Input: part model. Units: mm. Frame: model coordinates. Face numbers are marked on the shaded views. A direction names the side the tool comes from. Coordinates: 2 decimals unless noted, no trailing zeros. Write each loop counter-clockwise with the first axis right and the second up, starting at its lowest first coordinate (ties: lowest second). Pieces come first, ordered by that corner, then holes. Notation, with made-up numbers: M 8.5,67 L 19.5,67 A23 cw 19.5,97 Z; hole C -21.75,75 d2. An arc over 180 degrees is marked long. Use one line per item in the form item = value.
Solid Edge part; units mm, degrees
sketch "Sketch1" plane through (0, 0, 0) normal (0, 0, 1) x (1, 0, 0)
  arc A0 (60, 30) -> (60, -30) centre (60, 0) cw
  line L0 (0, -30) -> (60, -30)
  line L1 (-60, -30) -> (0, -30)
  arc A1 (-60, -30) -> (-60, 30) centre (-60, 0) cw
  line L2 (-60, 30) -> (0, 30)
  line L3 (0, 30) -> (60, 30)
  arc A2 (60, 15) -> (60, -15) centre (60, 0) cw
  line L4 (0, -15) -> (60, -15)
  line L5 (-60, -15) -> (0, -15)
  arc A3 (-60, -15) -> (-60, 15) centre (-60, 0) cw
  line L6 (-60, 15) -> (0, 15)
  line L7 (0, 15) -> (60, 15)
extrude "ExtrudedProtrusion_1" add sketch "Sketch1" along normal blind 20
sketch "Sketch2" plane through (0, 30, 10) normal (0, 1, 0) x (-1, 0, 0)
  circle A0 centre (0, 0) radius 5
extrude "ExtrudedProtrusion_2" add sketch "Sketch2" along normal blind 197
mirror "Mirror1" about plane through (0, 0, 10) normal (0, 1, 0) of "ExtrudedProtrusion_2"
sketch "Sketch3" plane through (0, -227, 10) normal (0, -1, 0) x (0, 0, -1)
  circle A0 centre (0, 0) radius 20
extrude "ExtrudedProtrusion_3" add sketch "Sketch3" along normal blind 40
mirror "Mirror2" about plane through (0, 0, 0) normal (0, -1, 0) of "ExtrudedProtrusion_3"
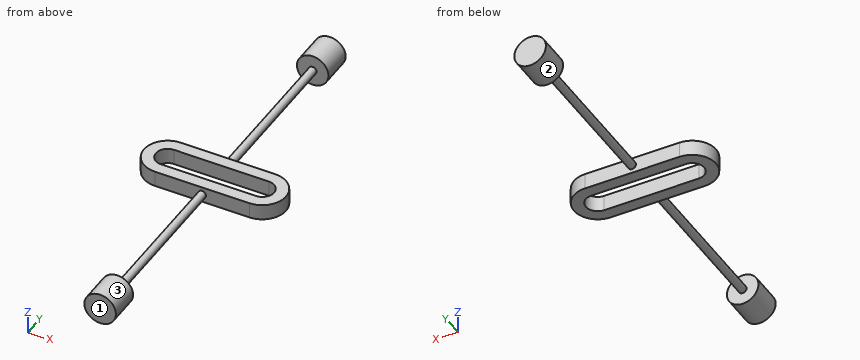
(1) Line query: probe 1 along Y at (x, z) = (10, 26); probe 2 along Y at (x, z) = (8.5, 0.5); probe 3 along Y at (x, z) = (52, 8). Output: solid intervals per line, ascending.
Computed:
probe_1 = -267 to -227, 227 to 267
probe_2 = -267 to -227, -30 to -15, 15 to 30, 227 to 267
probe_3 = -30 to -15, 15 to 30
(2) First-contact query: pin 1 Ø5 at (y, z) = (-152.5, 4.5) entering from -X; pin 2 Ø6 at (x, z) = (-24, 8.5) entering from -Y; pin 3 Ø10 at (x, z) = (21, 6.5) entering from +Y; pin 4 Ø1.5 at (x, z) = (-52.5, 17.5) entering from +Y. Flat tips, straight axial feed; report the tip coordinate or a pass-through.
Computed:
pin_1 = -4
pin_2 = -30
pin_3 = 267
pin_4 = 30
(3) Section query B-B on y = 0. Return the cut outline in (x, z), plus the area to 3 significant figures.
Computed:
outline = M -90,0 L -75,0 L -75,20 L -90,20 Z; M 75,0 L 90,0 L 90,20 L 75,20 Z
area = 600 mm^2
(4) Section query C-C on x = -38. Return the cut outline in (y, z).
Computed:
outline = M -30,0 L -15,0 L -15,20 L -30,20 Z; M 15,0 L 30,0 L 30,20 L 15,20 Z
(5) Section query A-A on x = 0. Return the cut outline in (y, z).
Computed:
outline = M -267,-10 L -227,-10 L -227,5 L -30,5 L -30,0 L -15,0 L -15,20 L -30,20 L -30,15 L -227,15 L -227,30 L -267,30 Z; M 15,0 L 30,0 L 30,5 L 227,5 L 227,-10 L 267,-10 L 267,30 L 227,30 L 227,15 L 30,15 L 30,20 L 15,20 Z
(6) Section query D-D on y = 69.5. Return the cut outline in (x, z).
Computed:
outline = C 0,10 d10
(7) Set-up query: the marked faces 1, 2 and 3. Return all of +Z, -Z, +X, -X, +Y, -Y with unobstructed straight access to the full face (end or side cutting, diameter ignored); none if empty.
Computed:
face_1 = +Z, -Z, +X, -X, -Y
face_2 = +Y
face_3 = -Y
